Could you check a few things on this model? Use its own coordinates, in mm. A direction names the side the tool comes from. Coordinates: 2 decimals unless noted, no trailing zeros. Loops run counter-clockwise (first coordinate to the right, second up) from the corner with the lowest first, then second, coordinate; pieces in that order, holes last.
1) Thinking about a two-plate mould opening in Z: for faces 5 (the face through (12, 59.428, 7)), 6 (the face through (-14, 61, 15)), 7 (the face through (-12.24, 62.22, 5.97)), 8 (the face through (-44.187, -2, 20)), which applies, released by +Z, released by -Z, zero draft, split by the parting line, or undercut?
2) For faces 1 (the face through (12.76, 62.22, 5.97)), 2 (the face through (29, -5.072, 15)), 3 (the face through (-44.687, 23, 8)), 4 (the face through (-30, 16, 0)), which set-ups out of +Z, -Z, +X, -X, +Y, -Y let a thin tool reach every point of the face, with its end or its side?
3) Imagine slicing it at B-B on z = 12.5. Please give me the cut outline in (x, y).
4) If I drill on line 1 along X through (y, z) = (62, 7); line 2 along Z through (x, y) = (-45, 22.5); line 3 along Y through (x, z) = (20.5, 4), over which ranges is the centre line in solid material (lowest first)?
5) Imagine slicing it at D-D on y = 18. Please give me the cut outline in (x, z), plus the area to 3 significant figures.
6) Will these pins go through, and if not, where does the flat tip stop? P1, Ø15, axis at y = 38.5, z = 21, coming from the +X side; P2, Ø12, axis at x = -23.5, y = 1.5, coming from the -Z side; P3, Ø16, axis at y = -3, z = 22.5, coming from the -X side; P4, Ø11, axis at y = -30, z = 4, coming from the +X side.
7) Imagine slicing it at C-C on x = -62. Please give me the cut outline in (y, z), plus the area to 3 significant figures.
```python
from build123d import *

# Parameters (mm, degrees)
SKETCH1_W                = 93
SKETCH1_H                = 100
BOSS_EXTRUDE2_DEPTH      = 10
SKETCH4_W                = 10.01
SKETCH4_H                = 15
BOSS_EXTRUDE4_DEPTH      = 24
SKETCH5_R                = 2
CUT_EXTRUDE1_DEPTH       = 50
SKETCH7_R                = 11
CUT_EXTRUDE3_DEPTH       = 50
SKETCH14_W               = 61.5
SKETCH14_H               = 42
CUT_EXTRUDE8_DEPTH       = 4
BOSS_EXTRUDE5_START      = -4
SKETCH16_W               = 61
SKETCH16_H               = 7.6
BOSS_EXTRUDE5_DEPTH      = 9
BOSS_EXTRUDE6_DEPTH      = 20
SKETCH19_R               = 11
CUT_EXTRUDE11_DEPTH      = 15
SKETCH20_R               = 2
CUT_EXTRUDE12_DEPTH      = 10
SKETCH8_R                = 1.4
CUT_EXTRUDE4_DEPTH       = 5.5
CUT_EXTRUDE13_DEPTH      = 103.078985596
CUT_EXTRUDE13_DEPTH_BACK = 103.078985596
SKETCH6_R                = 7.5


# Read off the part's stored shape, not the designer's step: Boss-Extrude6
with BuildPart() as part:
    # Sketch1 → Boss-Extrude2 (new body)
    with BuildSketch(Plane.XY):
        with Locations((-29.68705036, 14.928057554)):
            Rectangle(SKETCH1_W, SKETCH1_H)
    extrude(amount=BOSS_EXTRUDE2_DEPTH)

    # Sketch4 → Boss-Extrude4 (add)
    with BuildSketch(Plane(origin=(16.81294964, 0, 0), x_dir=(0, 0, -1), z_dir=(1, 0, 0))):
        with Locations((-4.995, -12.571942446)):
            Rectangle(SKETCH4_W, SKETCH4_H)
    extrude(amount=BOSS_EXTRUDE4_DEPTH)

    # Sketch5 → Cut-Extrude1 (cut)
    with BuildSketch(Plane(origin=(0, -5.071942446, 0), x_dir=(1, 0, 0), z_dir=(0, 1, 0))):
        with Locations(Location((26.81294964, -5, 0), (0, 0, 180))):
            Circle(SKETCH5_R)
    extrude(amount=-CUT_EXTRUDE1_DEPTH, mode=Mode.SUBTRACT)

    # Sketch7 → Cut-Extrude3 (cut)
    with BuildSketch(Plane(origin=(0, 0, 0), x_dir=(-1, 0, 0), z_dir=(0, 0, -1))):
        with Locations((24.18705036, 36.928057554)):
            Circle(SKETCH7_R)
    extrude(amount=-CUT_EXTRUDE3_DEPTH, mode=Mode.SUBTRACT)

    # Sketch14 → Cut-Extrude8 (cut)
    with BuildSketch(Plane.XY.offset(10)):
        with Locations((-13.93705036, 36.789132279)):
            Rectangle(SKETCH14_W, SKETCH14_H)
    extrude(amount=-CUT_EXTRUDE8_DEPTH, mode=Mode.SUBTRACT)

    # Sketch16 → Boss-Extrude5 (add)
    with BuildSketch(Plane.XY.offset(10).offset(BOSS_EXTRUDE5_START)):
        with Locations((-13.68705036, 61.128057554)):
            Rectangle(SKETCH16_W, SKETCH16_H)
    extrude(amount=BOSS_EXTRUDE5_DEPTH)

    # Boss-Extrude6 outline → Boss-Extrude6 (add)
    with BuildSketch(Plane.XY.offset(10)):
        Polygon((40.81294964, -5.071942446), (16.81294964, -5.071942446), (16.81294964, 15.789132279), (-44.18705036, 15.789132279), (-44.18705036, -20.071942446), (40.81294964, -20.071942446), align=None)
    extrude(amount=BOSS_EXTRUDE6_DEPTH)

    # Sketch19 → Cut-Extrude11 (cut)
    with BuildSketch(Plane(origin=(0, 0, 0), x_dir=(-1, 0, 0), z_dir=(0, 0, -1))):
        with Locations((53.18705036, 36.928057554)):
            Circle(SKETCH19_R)
    extrude(amount=-CUT_EXTRUDE11_DEPTH, mode=Mode.SUBTRACT)

    # Sketch20 → Cut-Extrude12 (cut)
    with BuildSketch(Plane.XY.offset(6)):
        with Locations((-34.68705036, 50.928057554)):
            Circle(SKETCH20_R)
        with Locations((5.31294964, 50.928057554)):
            Circle(SKETCH20_R)
        with Locations((-34.68705036, 22.928057554)):
            Circle(SKETCH20_R)
        with Locations((5.31294964, 22.928057554)):
            Circle(SKETCH20_R)
    extrude(amount=-CUT_EXTRUDE12_DEPTH, mode=Mode.SUBTRACT)

    # Sketch8 → Cut-Extrude4 (cut)
    with BuildSketch(Plane(origin=(0, 64.928057554, 0), x_dir=(1, 0, 0), z_dir=(0, 1, 0))):
        with Locations(Location((-13.18705036, -7, 0), (0, 0, 270))):
            Circle(SKETCH8_R)
        with Locations(Location((11.81294964, -7, 0), (0, 0, 270))):
            Circle(SKETCH8_R)
    extrude(amount=-CUT_EXTRUDE4_DEPTH, mode=Mode.SUBTRACT)

    # Sketch6 → Cut-Extrude13 (cut, two sides: drawn at the far end of the back side and taken through both)
    with BuildSketch(Plane(origin=(0, 0, 10), x_dir=(-1, 0, 0), z_dir=(0, 0, -1)).offset(-CUT_EXTRUDE13_DEPTH_BACK)):
        with Locations(Location((-1.81294964, -24.571942446, 0), (0, 0, 180))):
            Circle(SKETCH6_R)
    extrude(amount=CUT_EXTRUDE13_DEPTH + CUT_EXTRUDE13_DEPTH_BACK, mode=Mode.SUBTRACT)


solid = part.part
```
Filled in:
1. face 5: undercut
1. face 6: released by +Z
1. face 7: undercut
1. face 8: zero draft
2. face 1: +Y
2. face 2: +Z, -Z, +X, +Y
2. face 3: +Z, +X
2. face 4: -Z, +X, -X, +Y, -Y
3. outline: (-44.19, -20.07) - (-4.19, -20.07) arc R7.5 cw to (7.81, -20.07) - (40.81, -20.07) - (40.81, -5.07) - (16.81, -5.07) - (16.81, 15.79) - (-44.19, 15.79) - close; (-44.19, 57.33) - (16.81, 57.33) - (16.81, 64.93) - (-44.19, 64.93) - close
4. line 1: x = -76.19 to -14.59, -11.79 to 10.41, 13.21 to 16.81
4. line 2: z = 0 to 10
4. line 3: y = -20.07 to -5.07
5. outline: (-76.19, 0) - (16.81, 0) - (16.81, 6) - (-44.69, 6) - (-44.69, 10) - (-76.19, 10) - close
5. area: 684 mm2
6. P1: passes through
6. P2: stops at z = 0
6. P3: stops at x = -44.19
6. P4: stops at x = 16.81
7. outline: (-35.07, 0) - (30.35, 0) - (30.35, 10) - (-35.07, 10) - close; (43.51, 0) - (64.93, 0) - (64.93, 10) - (43.51, 10) - close
7. area: 868 mm2
